Geometry check sheet. Reference: the model listing, model coordinates, mm. Face numbers are marked on the shaded views. A direction names the side the tool comes from. Give positions to 0.01 mm unless a question says otherwise; leave off trailing zeros. Order: outer loops, then holes, each group sorted by start corner. A loop starts at its lowest first (then second) coordinate and runs counter-clockwise, first axis right, second up.
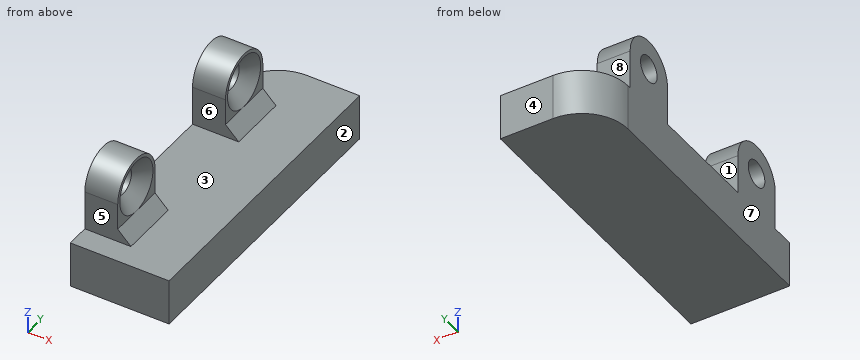
from build123d import *

# Parameters (mm, degrees)
BOSS_EXTRUDE1_DEPTH = 7
SKETCH2_R           = 2
BOSS_EXTRUDE2_DEPTH = 5
CHAMFER1_SIZE       = 2
CHAMFER2_SIZE       = 2


with BuildPart() as part:
    # Sketch1 → Boss-Extrude1 (new body)
    with BuildSketch(Plane.XY):
        with BuildLine():
            Line((22, 21), (14, 21))
            ThreePointArc((14, 21), (9.050252532, 18.949747468), (7, 14))
            Line((7, 14), (7, -25))
            Line((7, -25), (22, -25))
            Line((22, -25), (22, 21))
        make_face()
    extrude(amount=BOSS_EXTRUDE1_DEPTH)

    # Sketch2 → Boss-Extrude2 (add)
    with BuildSketch(Plane.ZY.offset(-7)):
        with BuildLine():
            Line((7, 13.5), (13, 13.5))
            ThreePointArc((13, 13.5), (17.5, 9), (13, 4.5))
            Line((13, 4.5), (7, 4.5))
            Line((7, 4.5), (7, 13.5))
        make_face()
        with Locations(Location((13, 9, 0), (0, 0, 270))):
            Circle(SKETCH2_R, mode=Mode.SUBTRACT)
    boss_extrude2 = extrude(amount=-BOSS_EXTRUDE2_DEPTH)

    # Mirror1: Boss-Extrude2 across plane
    add(boss_extrude2.mirror(Plane.ZX.offset(-4)))

    # Chamfer1
    chamfer1_edges = [part.edges().sort_by_distance(p)[0] for p in [
        (12, 11, 13),
        (12, -19, 13),
    ]]
    chamfer(chamfer1_edges, length=CHAMFER1_SIZE)

    # Chamfer2
    chamfer2_edges = [part.edges().sort_by_distance(p)[0] for p in [
        (12, 9, 7),
        (12, -17, 7),
    ]]
    chamfer(chamfer2_edges, length=CHAMFER2_SIZE - 0.0001)  # a hair under: the kernel refuses the full size


solid = part.part
Item 1: Sectioned sample at B-B (z = 8.5). Enter the section's corners in (x, y), and give its area (3 significant figures).
Reported:
outline: (7, -21.5) - (12.5, -21.5) - (12.5, -12.5) - (7, -12.5) - close; (7, 4.5) - (12.5, 4.5) - (12.5, 13.5) - (7, 13.5) - close
area: 99.0 mm2
Item 2: Set-up check for the marked faces 5, 6, 7 and 8: record each of +Z, -Z, +X, -X, +Y, -Y from which the full face is reachable in a straight line by a thin tool's end or side.
Reported:
face 5: +Z, +X, -X, -Y
face 6: +Z, +X, -X
face 7: +Z, -Z, -X, +Y, -Y
face 8: +Z, +X, -X, +Y
Item 3: Scan lines: L1, parallel to Y at x = 8, z = 7.75; L2, parallel to Z at x = 8.5, y = 9; L3, parallel to Z at x = 13, y = 1. Record each from-to range of solid material in increasing order.
Reported:
L1: y = -21.5 to -12.5, 4.5 to 13.5
L2: z = 0 to 11, 15 to 17.5
L3: z = 0 to 7
Item 4: Draft check along Y on the marked faces 1, 2, 3 and 4. Enter one of: released by +Y, released by -Y, zero draft, split by the parting line, or undercut.
Reported:
face 1: undercut
face 2: zero draft
face 3: undercut
face 4: released by +Y
Item 5: Sectioned sample at D-D (x = 17.75). Enter the section's corners in (y, z), and give its area (3 significant figures).
Reported:
outline: (-25, 0) - (21, 0) - (21, 7) - (-25, 7) - close
area: 322 mm2
Item 6: Gauge pin test, flat ends, axial feed: pin 1 (5 mm diameter, centred on x = 11.5, z = 10.5, fed in from +Y); pin 2 (9.5 mm diameter, centred on y = 8, z = 14, fed in from +X); pin 3 (1.8 mm diameter, centred on x = 9.5, z = 9, fed in from -Y). Record the tip position at first contact, or that the pin passes through.
Reported:
pin 1: stops at y = 13.5
pin 2: stops at x = 12
pin 3: stops at y = -21.5
Item 7: Sectioned sample at C-C (z = 2.5). Enter the section's corners in (x, y), and give its area (3 significant figures).
Reported:
outline: (7, -25) - (22, -25) - (22, 21) - (14, 21) arc R7 ccw to (7, 14) - close
area: 679 mm2
